Verification items for the finished model (mm, model axes). A direction names the side the tool comes from. Coordinates: 2 decimals unless noted, no trailing zeros. Write each loop counter-clockwise with the first axis right and the second up, starting at its lowest first coordinate (ties: lowest second). Pieces come first, ordered by that corner, then holes.
```python
from build123d import *

# Parameters (mm, degrees)
SKETCH_1_R      = 7
SKETCH_1_R_2    = 2
EXTRUDE_1_DEPTH = 100


with BuildPart() as part:
    # 草图1 → 凸台-拉伸1 (new body)
    with BuildSketch(Plane.XY):
        with BuildLine():
            Line((-16.096789658, 15.945460798), (-16.096789658, 16.045460798))
            ThreePointArc((-16.096789658, 16.045460798), (-16.653286773, 17.388963682), (-17.996789658, 17.945460798))
            Line((-17.996789658, 17.945460798), (-27.596789658, 17.945460798))
            ThreePointArc((-27.596789658, 17.945460798), (-28.303896439, 17.652567579), (-28.596789658, 16.945460798))
            Line((-28.596789658, 16.945460798), (-28.596789658, 7.345460798))
            ThreePointArc((-28.596789658, 7.345460798), (-28.040292542, 6.001957914), (-26.696789658, 5.445460798))
            Line((-26.696789658, 5.445460798), (-26.596789658, 5.445460798))
            Line((-26.596789658, 5.445460798), (-26.596789658, 10.445460798))
            Line((-26.596789658, 10.445460798), (-22.864556611, 10.445460798))
            Line((-22.864556611, 10.445460798), (-20.096789658, 7.677693845))
            Line((-20.096789658, 7.677693845), (-20.096789658, -6.786772249))
            Line((-20.096789658, -6.786772249), (-22.864556611, -9.554539202))
            Line((-22.864556611, -9.554539202), (-26.596789658, -9.554539202))
            Line((-26.596789658, -9.554539202), (-26.596789658, -4.554539202))
            Line((-26.596789658, -4.554539202), (-26.696789658, -4.554539202))
            ThreePointArc((-26.696789658, -4.554539202), (-28.040292542, -5.111036318), (-28.596789658, -6.454539202))
            Line((-28.596789658, -6.454539202), (-28.596789658, -16.054539202))
            ThreePointArc((-28.596789658, -16.054539202), (-28.303896439, -16.761645983), (-27.596789658, -17.054539202))
            Line((-27.596789658, -17.054539202), (-17.996789658, -17.054539202))
            ThreePointArc((-17.996789658, -17.054539202), (-16.653286773, -16.498042086), (-16.096789658, -15.154539202))
            Line((-16.096789658, -15.154539202), (-16.096789658, -15.054539202))
            Line((-16.096789658, -15.054539202), (-21.096789658, -15.054539202))
            Line((-21.096789658, -15.054539202), (-21.096789658, -11.322306155))
            Line((-21.096789658, -11.322306155), (-18.329022705, -8.554539202))
            Line((-18.329022705, -8.554539202), (-3.864556611, -8.554539202))
            Line((-3.864556611, -8.554539202), (-1.096789658, -11.322306155))
            Line((-1.096789658, -11.322306155), (-1.096789658, -15.054539202))
            Line((-1.096789658, -15.054539202), (-6.096789658, -15.054539202))
            Line((-6.096789658, -15.054539202), (-6.096789658, -15.154539202))
            ThreePointArc((-6.096789658, -15.154539202), (-5.540292542, -16.498042086), (-4.196789658, -17.054539202))
            Line((-4.196789658, -17.054539202), (5.403210342, -17.054539202))
            ThreePointArc((5.403210342, -17.054539202), (6.110317124, -16.761645983), (6.403210342, -16.054539202))
            Line((6.403210342, -16.054539202), (6.403210342, -6.454539202))
            ThreePointArc((6.403210342, -6.454539202), (5.846713227, -5.111036318), (4.503210342, -4.554539202))
            Line((4.503210342, -4.554539202), (4.403210342, -4.554539202))
            Line((4.403210342, -4.554539202), (4.403210342, -9.554539202))
            Line((4.403210342, -9.554539202), (0.670977295, -9.554539202))
            Line((0.670977295, -9.554539202), (-2.096789658, -6.786772249))
            Line((-2.096789658, -6.786772249), (-2.096789658, 7.677693845))
            Line((-2.096789658, 7.677693845), (0.670977295, 10.445460798))
            Line((0.670977295, 10.445460798), (4.403210342, 10.445460798))
            Line((4.403210342, 10.445460798), (4.403210342, 5.445460798))
            Line((4.403210342, 5.445460798), (4.503210342, 5.445460798))
            ThreePointArc((4.503210342, 5.445460798), (5.846713227, 6.001957914), (6.403210342, 7.345460798))
            Line((6.403210342, 7.345460798), (6.403210342, 16.945460798))
            ThreePointArc((6.403210342, 16.945460798), (6.110317124, 17.652567579), (5.403210342, 17.945460798))
            Line((5.403210342, 17.945460798), (-4.196789658, 17.945460798))
            ThreePointArc((-4.196789658, 17.945460798), (-5.540292542, 17.388963682), (-6.096789658, 16.045460798))
            Line((-6.096789658, 16.045460798), (-6.096789658, 15.945460798))
            Line((-6.096789658, 15.945460798), (-1.096789658, 15.945460798))
            Line((-1.096789658, 15.945460798), (-1.096789658, 12.213227751))
            Line((-1.096789658, 12.213227751), (-3.864556611, 9.445460798))
            Line((-3.864556611, 9.445460798), (-18.329022705, 9.445460798))
            Line((-18.329022705, 9.445460798), (-21.096789658, 12.213227751))
            Line((-21.096789658, 12.213227751), (-21.096789658, 15.945460798))
            Line((-21.096789658, 15.945460798), (-16.096789658, 15.945460798))
        make_face()
        with Locations((-11.096789658, 0.445460798)):
            Circle(SKETCH_1_R, mode=Mode.SUBTRACT)
        with Locations((-24.846789658, 14.195460798)):
            Circle(SKETCH_1_R_2, mode=Mode.SUBTRACT)
        with Locations((2.653210342, 14.195460798)):
            Circle(SKETCH_1_R_2, mode=Mode.SUBTRACT)
        with Locations((-24.846789658, -13.304539202)):
            Circle(SKETCH_1_R_2, mode=Mode.SUBTRACT)
        with Locations((2.653210342, -13.304539202)):
            Circle(SKETCH_1_R_2, mode=Mode.SUBTRACT)
    extrude(amount=EXTRUDE_1_DEPTH)


solid = part.part
```
1. Gauge pin test, flat ends, axial feed: P1, Ø5.5, axis at x = -4.5, z = 57.5, coming from the -Y side; P2, Ø8, axis at x = -11.5, z = 39.5, coming from the -Y side; P3, Ø4, axis at x = -11, z = 23, coming from the +Y side; P4, Ø7, axis at y = 1.5, z = 44.5, coming from the +X side. Record the tip position at first contact, or that the pin passes through.
2. Tool access check on faces 5 (the cylindrical face through (-28.055, 6.017, 49.3)), 6 (the flat face through (-23, -17.055, 49)), 7 (the flat face through (-25, 10.445, 49)). Record the directions out of +Z, -Z, +X, -X, +Y, -Y that give a thin tool (end or side, any length) a straight path to the whole face; none if there is none.
3. Sectioned sample at C-C, the plane z = 25. Give the number of separate pieces and of enclosed holes in the cut face, and give its area (3 significant figures).
4. Draft check along Y on faces 1 (the flat face through (-23, 17.945, 49)), 2 (the flat face through (-11, 8, 100)), 3 (the flat face through (1, -17.055, 49)), 4 (the flat face through (-4, -15.055, 49)). Enter one of: pulls with the +Y half, pulls with the -Y half, needs draft (parallel to the pull), parting line crosses it, or undercut.
5. Material ranges on L1, parallel to Y at x = 2.5, z = 5; L2, parallel to X at y = 15.5, z = 23; L3, parallel to X at y = -9.5, z = 81.5, recorded low to high.
6. Sectioned sample at B-B, the plane y = 3. Record the boundary of the cut face in (x, z).
7. Sectioned sample at A-A, the plane x = -13. Record the boundary of the cut face in (y, z).
Outcome:
1. P1: stops at y = -17.05
1. P2: stops at y = -8.55
1. P3: stops at y = 9.45
1. P4: stops at x = -2.1
2. face 5: +Z, -Z, -X
2. face 6: +Z, -Z, +X, -X, -Y
2. face 7: +Z, -Z
3. separate pieces: 1
3. enclosed holes: 5
3. area: 444 mm2
4. face 1: pulls with the +Y half
4. face 2: needs draft
4. face 3: pulls with the -Y half
4. face 4: undercut
5. L1: y = -17.05 to -15.3, -11.31 to -9.55, 10.45 to 12.2, 16.19 to 17.95
5. L2: x = -28.6 to -26.36, -23.33 to -21.1, -1.1 to 1.14, 4.17 to 6.4
5. L3: x = -28.6 to -26.6, -22.81 to -19.27, -2.92 to 0.62, 4.4 to 6.4
6. outline: (-20.1, 0) - (-17.61, 0) - (-17.61, 100) - (-20.1, 100) - close; (-4.58, 0) - (-2.1, 0) - (-2.1, 100) - (-4.58, 100) - close
7. outline: (-8.55, 0) - (-6.29, 0) - (-6.29, 100) - (-8.55, 100) - close; (7.18, 0) - (9.45, 0) - (9.45, 100) - (7.18, 100) - close
